For this review, take the finished solid that the model builds, in its own axes (mm). Face numbers are marked on the shaded views. A direction names the side the tool comes from. Round coordinates to 2 decimals unless told otherwise and drop trailing zeros. Write each loop counter-clockwise with the first axis right and the second up, starting at its lowest first coordinate (ties: lowest second). Pieces come first, ordered by that corner, then holes. Notation, with made-up numbers: (49, 65) -> (81, 65) arc R26 ccw to (81, 102) -> close; hole circle Ø3 at (-19, 57.25). An arc over 180 degrees is marked (long way). Answer in a Markdown table with one row per item.
from build123d import *

# Parameters (mm, degrees)
BASESTEELANGLE_DEPTH                             = 44.45
F_3_8_16_TAPPED_HOLE1_D                          = 7.9375
CBORE_FOR_10_SOCKET_HEAD_CAP_SCREW2_D            = 5.1054
CBORE_FOR_10_SOCKET_HEAD_CAP_SCREW2_CBORE_D      = 9.525
CBORE_FOR_10_SOCKET_HEAD_CAP_SCREW2_CBORE_DEPTH  = 4.826
SKETCH16_W                                       = 94.308892356
SKETCH16_H                                       = 144.501300052
CUT_EXTRUDE1_DEPTH                               = 25.4
F_10_32_TAPPED_HOLE3_D                           = 4.0386
F_10_32_TAPPED_HOLE3_DEPTH                       = 13.6144
F_10_32_TAPPED_HOLE3_TIP                         = 1.213317848
F_10_32_TAPPED_HOLE4_D                           = 4.0386
F_10_32_TAPPED_HOLE4_DEPTH                       = 13.6144
F_10_32_TAPPED_HOLE4_TIP                         = 1.213317848
CBORE_FOR_1_4_SOCKET_HEAD_CAP_SCREW1_D           = 6.7564
CBORE_FOR_1_4_SOCKET_HEAD_CAP_SCREW1_CBORE_D     = 11.1125
CBORE_FOR_1_4_SOCKET_HEAD_CAP_SCREW1_CBORE_DEPTH = 6.35
SKETCH19_R                                       = 25.4
CUT_EXTRUDE2_DEPTH                               = 0.508
CHAMFER1_SIZE                                    = 2.54


with BuildPart() as part:
    # Sketch1 → BaseSteelAngle (new body, symmetric)
    with BuildSketch(Plane.XY):
        with BuildLine():
            Line((0, 0), (0, 152.4))
            Line((0, 152.4), (6.35508, 152.4))
            ThreePointArc((6.35508, 152.4), (13.086679988, 149.611679988), (15.875, 142.88008))
            Line((15.875, 142.88008), (15.875, 28.575))
            ThreePointArc((15.875, 28.575), (19.594743879, 19.594743879), (28.575, 15.875))
            Line((28.575, 15.875), (142.88008, 15.875))
            ThreePointArc((142.88008, 15.875), (149.611679988, 13.086679988), (152.4, 6.35508))
            Line((152.4, 6.35508), (152.4, 0))
            Line((152.4, 0), (0, 0))
        make_face()
    extrude(amount=BASESTEELANGLE_DEPTH, both=True)

    # 3/8-16 Tapped Hole1 (through all)
    with Locations(Plane.ZY):
        with Locations((0, 112.8903)):
            Hole(F_3_8_16_TAPPED_HOLE1_D / 2)

    # CBORE for #10 Socket Head Cap Screw2 (through all)
    with Locations(Plane(origin=(15.875, 58.160616164, 30.43670953), x_dir=(0, 0, 1), z_dir=(1, 0, 0))):
        with Locations((-46.31170953, -0.259383836), (-14.56170953, -0.259383836), (-14.56170953, -76.459383836), (-46.31170953, -76.459383836)):
            CounterBoreHole(CBORE_FOR_10_SOCKET_HEAD_CAP_SCREW2_D / 2, CBORE_FOR_10_SOCKET_HEAD_CAP_SCREW2_CBORE_D / 2, CBORE_FOR_10_SOCKET_HEAD_CAP_SCREW2_CBORE_DEPTH)

    # Sketch16 → Cut-Extrude1 (cut, symmetric)
    with BuildSketch(Plane(origin=(0, 0, 0), x_dir=(1, 0, 0), z_dir=(0, 1, 0))):
        with Locations((136.054446178, 1.452938118)):
            Rectangle(SKETCH16_W, SKETCH16_H)
    extrude(amount=CUT_EXTRUDE1_DEPTH, both=True, mode=Mode.SUBTRACT)

    # #10-32 Tapped Hole3
    with Locations(Plane.ZY):
        with Locations((-31.75, 82.55), (31.75, 82.55), (31.75, 19.05), (-31.75, 19.05)):
            Hole(F_10_32_TAPPED_HOLE3_D / 2, depth=F_10_32_TAPPED_HOLE3_DEPTH)
            with Locations((0, 0, -(F_10_32_TAPPED_HOLE3_DEPTH + F_10_32_TAPPED_HOLE3_TIP / 2))):  # 118° drill point
                Cone(0, F_10_32_TAPPED_HOLE3_D / 2, F_10_32_TAPPED_HOLE3_TIP, mode=Mode.SUBTRACT)

    # #10-32 Tapped Hole4
    with Locations(Plane.XZ):
        with Locations((76.2, 31.75), (12.7, 31.75), (12.7, -31.75), (76.2, -31.75)):
            Hole(F_10_32_TAPPED_HOLE4_D / 2, depth=F_10_32_TAPPED_HOLE4_DEPTH)
            with Locations((0, 0, -(F_10_32_TAPPED_HOLE4_DEPTH + F_10_32_TAPPED_HOLE4_TIP / 2))):  # 118° drill point
                Cone(0, F_10_32_TAPPED_HOLE4_D / 2, F_10_32_TAPPED_HOLE4_TIP, mode=Mode.SUBTRACT)

    # CBORE for 1/4 Socket Head Cap Screw1 (through all)
    with Locations(Plane(origin=(0, 15.875, 0), x_dir=(-1, 0, 0), z_dir=(0, 1, 0))):
        with Locations((-44.45, 0)):
            CounterBoreHole(CBORE_FOR_1_4_SOCKET_HEAD_CAP_SCREW1_D / 2, CBORE_FOR_1_4_SOCKET_HEAD_CAP_SCREW1_CBORE_D / 2, CBORE_FOR_1_4_SOCKET_HEAD_CAP_SCREW1_CBORE_DEPTH)

    # Sketch19 → Cut-Extrude2 (cut)
    with BuildSketch(Plane.XZ):
        with Locations((44.45, 0)):
            Circle(SKETCH19_R)
    extrude(amount=-CUT_EXTRUDE2_DEPTH, mode=Mode.SUBTRACT)

    # Chamfer1
    chamfer1_edges = [part.edges().sort_by_distance(p)[0] for p in [
        (0, 76.2, 44.45),
        (88.9, 7.9375, -44.45),
        (88.9, 7.9375, 44.45),
        (88.9, 15.875, 0),
        (0, 76.2, -44.45),
    ]]
    chamfer(chamfer1_edges, length=CHAMFER1_SIZE)


solid = part.part
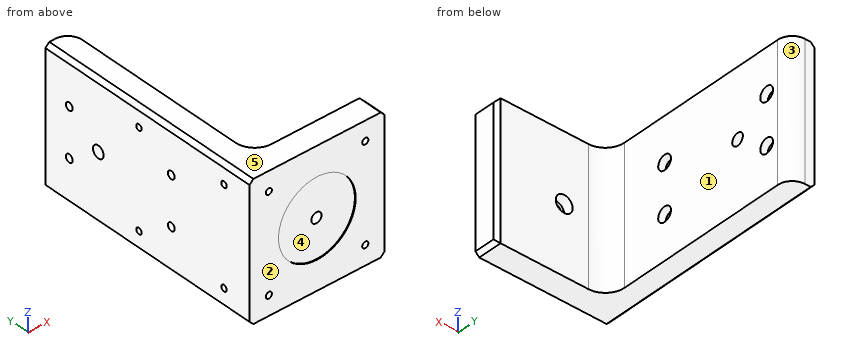
1) Consider section B-B on z = 0. State the section outline as (x, y) points (3 decimals).
Solved:
| item | result |
|---|---|
| outline | (0, 0) -> (19.05, 0) -> (19.05, 0.508) -> (41.072, 0.508) -> (41.072, 9.525) -> (38.894, 9.525) -> (38.894, 15.875) -> (28.575, 15.875) arc R12.7 cw to (15.875, 28.575) -> (15.875, 108.922) -> (0, 108.922) -> close; (0, 116.859) -> (15.875, 116.859) -> (15.875, 142.88) arc R9.52 ccw to (6.355, 152.4) -> (0, 152.4) -> close; (47.828, 0.508) -> (69.85, 0.508) -> (69.85, 0) -> (88.9, 0) -> (88.9, 13.335) -> (86.36, 15.875) -> (50.006, 15.875) -> (50.006, 9.525) -> (47.828, 9.525) -> close |
2) Consider section D-D on z = 36.5. State the section outline as (x, y) points (3 decimals).
Solved:
| item | result |
|---|---|
| outline | (0, 0) -> (88.9, 0) -> (88.9, 13.335) -> (86.36, 15.875) -> (28.575, 15.875) arc R12.7 cw to (15.875, 28.575) -> (15.875, 142.88) arc R9.52 ccw to (6.355, 152.4) -> (0, 152.4) -> close |
3) For the marked faces 1 and 2, list the 3-axis set-ups (+Z, -Z, +X, -X, +Y, -Y) from which the entire face can be reached by the end or side of a thin tool; tool diameter is ignored.
Solved:
| item | result |
|---|---|
| face 1 | +Z, -Z, +X, +Y |
| face 2 | +Z, -Z, +X, -X, -Y |
4) Clearance check with flat-ended pins moving along their axes: pin 1 Ø12 at (x, z) = (59, 10.5) entering from +Y (3 decimals); pin 2 Ø3 at (y, z) = (82.55, 31.75) entering from -X; pin 3 Ø1 at (x, z) = (55, -5.5) entering from -Y. State where each tip first meets the part, or that it passes through.
Solved:
| item | result |
|---|---|
| pin 1 | y = 15.875 |
| pin 2 | x = 13.93 |
| pin 3 | y = 0.51 |
5) Consider section A-A on y = 134.62. State how many separate pieces and enclosed holes the cut face has, then the cut area to 3 significant figures.
Solved:
| item | result |
|---|---|
| separate pieces | 3 |
| enclosed holes | 0 |
| area | 1,200 mm² |
6) Consider section C-C on x = 43.5. State the section outline as (y, z) points (3 decimals), then the cut area to 3 significant figures.
Solved:
| item | result |
|---|---|
| outline | (0, -44.45) -> (15.875, -44.45) -> (15.875, -5.474) -> (9.525, -5.474) -> (9.525, -3.242) -> (0.508, -3.242) -> (0.508, -25.382) -> (0, -25.382) -> close; (0, 25.382) -> (0.508, 25.382) -> (0.508, 3.242) -> (9.525, 3.242) -> (9.525, 5.474) -> (15.875, 5.474) -> (15.875, 44.45) -> (0, 44.45) -> close |
| area | 1,260 mm² |
7) Mouldability with a two-part tool opening along Z and no side actions: class the marked faces 3, 4 and 5 as pulls with the +Z half, pulls with the -Z half, needs draft (parallel to the pull), parting line crosses it, or undercut.
Solved:
| item | result |
|---|---|
| face 3 | needs draft |
| face 4 | undercut |
| face 5 | pulls with the +Z half |
8) For line 1 (Z direction, x = 5, y = 134.62); line 2 (Z direction, x = 13.95, y = 58.42); line 3 (Z direction, x = 44, y = 12), list the stretches that pass through material, from the lowest coordinate up. Write a range as [from, to].
Solved:
| item | result |
|---|---|
| line 1 | [-44.45, -18.43], [-13.32, 13.32], [18.43, 44.45] |
| line 2 | [-44.45, -20.64], [-11.11, 11.11], [20.64, 44.45] |
| line 3 | [-44.45, -5.54], [5.54, 44.45] |
